Could you check a few things on this model? Use its own coordinates, in mm. Face numbers are marked on the shaded views. A direction names the side the tool comes from. Round coordinates to 2 decimals unless told otherwise and drop trailing zeros. Write each loop counter-clockwise with the first axis right and the second up, starting at its lowest first coordinate (ties: lowest second). Pieces come first, ordered by that corner, then holes. Notation, with made-up numbers: (89, 8.5) -> (97, 8.5) arc R33 cw to (97, 44.5) -> close; hole circle Ø2 at (-33.5, -18). An arc over 180 degrees is marked (long way). Return JSON: item names as keys, results as strings.
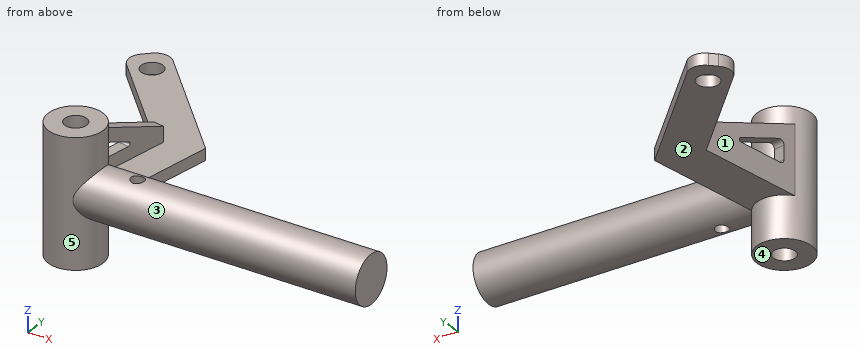
Solid Edge part; units mm, degrees
sketch "Sketch1" plane through (0, 0, 0) normal (0, 0, 1) x (1, 0, 0)
  circle A0 centre (0, 0) radius 12.5
extrude "Protrusion1" add sketch "Sketch1" along normal blind 58
sketch "Sketch2" plane through (0, 0, 0) normal (1, 0, 0) x (0, 1, 0)
  circle A0 centre (0, 30.6149) radius 11
extrude "ExtrudedProtrusion_2" add sketch "Sketch2" along normal blind 135
sketch "Sketch3" plane through (0, 0, 58) normal (0, 0, 1) x (1, 0, 0)
  circle A0 centre (0, 0) radius 5
extrude "ExtrudedCutout_1" cut sketch "Sketch3" against normal blind 74.8467
cosmetic_thread "Thread_1" thread depth 22
sketch "Sketch4" plane through (0, 0, 0) normal (0, 0, 1) x (1, 0, 0)
  circle A0 centre (28.334, 0) radius 3
extrude "ExtrudedCutout_2" cut sketch "Sketch4" along normal blind 57.1507
sketch "Sketch5" plane through (0, 0, 19.1008) normal (0, 0, 1) x (1, 0, 0)
  arc A0 (-10.1543, 6) -> (10.1543, 6) centre (0, 0) cw
  line L0 (19.7049, 60.1644) -> (10.1543, 6)
  line L1 (-28.5835, 110.8421) -> (19.7049, 60.1644)
  arc A1 (-38.4801, 111.0811) -> (-28.5835, 110.8421) centre (-33.6513, 106.0133) cw
  line L2 (-41.376, 108.3217) -> (-38.4801, 111.0811)
  arc A2 (-41.376, 108.3217) -> (-41.6149, 98.4251) centre (-36.5471, 103.2539) ccw
  line L3 (-1.3148, 56.131) -> (-41.6149, 98.4251)
  line L4 (-10.1543, 6) -> (-1.3148, 56.131)
  dimension "D1" = 28.5835
  dimension "D2" = 19.7049
  dimension "D3" = 28.5835
extrude "ExtrudedProtrusion_3" add sketch "Sketch5" along normal blind 5.3111
sketch "Sketch6" plane through (-15.6273, 67.3558, 24.4118) normal (0, 0, 1) x (-0.6898, 0.724, 0)
  circle A0 centre (35.4203, -11.6185) radius 5
extrude "ExtrudedCutout_5" cut sketch "Sketch6" against normal blind 21.5165 and the other way blind 19.734
sketch "Sketch7" plane through (-5.5858, 31.9091, 21.7563) normal (-0.9848, 0.1736, 0) x (-0.1736, -0.9848, 0)
  line L0 (24.5955, 2.6555) -> (-24.5955, 2.6555)
  line L1 (-24.5955, 2.6555) -> (-24.5955, 9.6555)
  line L2 (-24.5955, 9.6555) -> (24.5955, 28.6555)
  line L3 (24.5955, 28.6555) -> (24.5955, 2.6555)
  line L4 (-5.1676, 8.6555) -> (16.5955, 8.6555)
  arc A0 (16.5955, 8.6555) -> (18.5955, 10.6555) centre (16.5955, 10.6555) ccw
  line L5 (18.5955, 10.6555) -> (18.5955, 16.9895)
  arc A1 (15.8749, 18.8552) -> (18.5955, 16.9895) centre (16.5955, 16.9895) cw
  line L6 (15.8749, 18.8552) -> (-5.5279, 10.5884)
  arc A2 (-5.5279, 10.5884) -> (-5.1676, 8.6555) centre (-5.1676, 9.6555) ccw
  dimension "D1" = 24.5955
  dimension "D2" = 24.5955
extrude "ExtrudedProtrusion_5" add sketch "Sketch7" against normal blind 5
properties material "Steel"
1) I want a section at B-B, the plane z = 3.5. Please give me the cut outline in (x, y), and give its area (3 significant figures).
Return value:
{"outline": "circle Ø25 at (0, 0); hole circle Ø10 at (0, 0)", "area": "412 mm²"}
2) If I drill on probe 1 along Y at (x, z) = (0, 14); probe 2 along Y at (x, z) = (15, 31); probe 3 along X at (y, z) = (68, 19.5), over which ranges is the centre line in solid material (lowest first)? Write a range as [from, to].
Return value:
{"probe 1": "[-12.5, -5], [5, 12.5]", "probe 2": "[-10.99, 10.99]", "probe 3": "[-12.62, 12.24]"}
3) I want a section at D-D, the plane x = 114. Please give me the cut outline in (y, z), and give its area (3 significant figures).
Return value:
{"outline": "circle Ø22 at (0, 30.61)", "area": "380 mm²"}
4) I want a section at C-C, the plane y = 67. Please give me the cut outline in (x, z).
Return value:
{"outline": "(-11.67, 19.1) -> (13.19, 19.1) -> (13.19, 24.41) -> (-11.67, 24.41) -> close"}
5) Will these pins go through, and if not, where does the flat tip stop? pin 1 Ø4.5 at (x, y) = (-6, 28) entering from +Z; pin 2 Ø10 at (x, z) = (33, 27) entering from +Y; pin 3 Ø19 at (x, y) = (-14, 63) entering from -Z; pin 4 Ø5.5 at (x, y) = (28.334, 0) entering from +Z.
Return value:
{"pin 1": "z = 43.3", "pin 2": "y = 11", "pin 3": "z = 19.1", "pin 4": "through"}
6) I want a section at A-A, the plane y = 0. Please give me the cut outline in (x, z), and give its area (3 significant figures).
Return value:
{"outline": "(-12.5, 0) -> (-5, 0) -> (-5, 58) -> (-12.5, 58) -> close; (5, 0) -> (12.5, 0) -> (12.5, 19.61) -> (25.33, 19.61) -> (25.33, 41.61) -> (12.5, 41.61) -> (12.5, 58) -> (5, 58) -> close; (31.33, 19.61) -> (135, 19.61) -> (135, 41.61) -> (31.33, 41.61) -> close", "area": "3,430 mm²"}
7) Thinking about a two-plate mould opening in Y: for the marked faces 1 and 2, which applies, pulls with the +Y half, pulls with the -Y half, needs draft (parallel to the pull), parting line crosses it, or undercut?
Return value:
{"face 1": "undercut", "face 2": "needs draft"}
8) For the marked faces 3, 4 and 5, which set-ups out of +Z, -Z, +X, -X, +Y, -Y let a thin tool reach every point of the face, with its end or its side?
Return value:
{"face 3": "+X", "face 4": "-Z, +X, -X, +Y, -Y", "face 5": "none"}
